Part model, mm, in its own coordinate system. A direction names the side the tool comes from. Coordinates: 2 decimals unless noted, no trailing zeros. Write each loop counter-clockwise with the first axis right and the second up, starting at its lowest first coordinate (ties: lowest second). Pieces come first, ordered by that corner, then holes. Notation, with made-up numbers: (63.25, 10.5) -> (112.25, 10.5) arc R22 ccw to (112.25, 32.5) -> close; hole circle Ø10 at (47.5, -6.5). An arc over 180 degrees is marked (long way). Write item = value, one per line.
from build123d import *

# Parameters (mm, degrees)
CROQUIS1_R              = 1
SALIENTE_EXTRUIR1_DEPTH = 3


with BuildPart() as part:
    # Croquis1 → Saliente-Extruir1 (new body)
    with BuildSketch(Plane(origin=(0, 0, 0), x_dir=(1, 0, 0), z_dir=(0, 1, 0))):
        with BuildLine():
            Line((-1.930199007, 22.227708448), (9.995007766, -0.44472952))
            Line((9.995007766, -0.44472952), (9.995007766, -23.778062853))
            Line((9.995007766, -23.778062853), (14.995007766, -30.44472952))
            Line((14.995007766, -30.44472952), (19.995007766, -30.44472952))
            Line((19.995007766, -30.44472952), (19.995007766, -20.44472952))
            Line((19.995007766, -20.44472952), (14.995007766, -13.778062853))
            Line((14.995007766, -13.778062853), (14.995007766, -3.222172626))
            Line((14.995007766, -3.222172626), (17.495007766, 1.777827374))
            Line((17.495007766, 1.777827374), (17.495007766, 6.777827374))
            Line((17.495007766, 6.777827374), (6.920214539, 26.882832512))
            ThreePointArc((6.920214539, 26.882832512), (0.167445734, 28.980477254), (-1.930199007, 22.227708448))
        make_face()
        with Locations((2.495007766, 24.55527048)):
            Circle(CROQUIS1_R, mode=Mode.SUBTRACT)
        with Locations((12.371532383, 5.777827374)):
            Circle(CROQUIS1_R, mode=Mode.SUBTRACT)
    extrude(amount=SALIENTE_EXTRUIR1_DEPTH)


solid = part.part
Q1. Saw through at D-D on x = 4.75. Give the cut face in (y, z), and give its area (3 significant figures).
Model answer:
outline = (0, -29.02) -> (3, -29.02) -> (3, -9.53) -> (0, -9.53) -> close
area = 58.5 mm²
Q2. Mould opens along Z. For faces 1 (the face through (12.28, 1.48, -16.69)), 2 (the face through (14.995, 1, 9)), 3 (the face through (11, 0, 0)) say: released by +Z, released by -Z, zero draft, split by the parting line, or undercut.
Model answer:
face_1 = released by -Z
face_2 = undercut
face_3 = zero draft
Q3. Saw through at C-C on z = 7. Give the cut face in (x, y) (3 decimals), and give its area (3 significant figures).
Model answer:
outline = (9.995, 0) -> (14.995, 0) -> (14.995, 3) -> (9.995, 3) -> close
area = 15.0 mm²
Q4. Which spindle directions (+Z, -Z, +X, -X, +Y, -Y) get a long thin tool onto all of the face, cutting with end or side? Do faces 4 (the face through (17.495, 1, -4)), 5 (the face through (16.228, 1.479, 0.757)), 6 (the face through (9.995, 1, 12)). Say none if no direction does.
Model answer:
face_4 = -Z, +X, +Y, -Y
face_5 = +X, +Y, -Y
face_6 = +Z, -X, +Y, -Y
Q5. Saw through at B-B on y = 2.1. Give the cut face in (x, z) (3 decimals), and give its area (3 significant figures).
Model answer:
outline = (-1.93, -22.228) arc R5 ccw to (6.92, -26.883) -> (17.495, -6.778) -> (17.495, -1.778) -> (14.995, 3.222) -> (14.995, 13.778) -> (19.995, 20.445) -> (19.995, 30.445) -> (14.995, 30.445) -> (9.995, 23.778) -> (9.995, 0.445) -> close; hole circle Ø2 at (2.495, -24.555); hole circle Ø2 at (12.372, -5.778)
area = 502 mm²
Q6. Saw through at A-A on x = 12.75. Give the cut face in (y, z), and give its area (3 significant figures).
Model answer:
outline = (0, -15.8) -> (3, -15.8) -> (3, -6.7) -> (0, -6.7) -> close; (0, -4.85) -> (3, -4.85) -> (3, 27.45) -> (0, 27.45) -> close
area = 124 mm²
Q7. Pin check, flat tips, straight feed: pin 1 (0.9 mm diameter, centred on y = 2, z = 7, fed in from -X) (3 decimals); pin 2 (1.5 mm diameter, centred on x = 1, y = 1.5, fed in from +Z); pin 3 (1.5 mm diameter, centred on y = 2, z = 8, fed in from +X) (3 decimals). Stop position of each tip, or through.
Model answer:
pin_1 = 9.995
pin_2 = -15.23
pin_3 = 14.995
Q8. Probe line 1 (X direction, y = 0.65, z = 6) (3 decimals); line 2 (Z direction, x = 3.25, y = 0.85); line 3 (X direction, y = 1.9, z = -5) (3 decimals). List the from-to ranges inside material, lowest first. Write a range as from..to.
Model answer:
line_1 = 9.995..14.995
line_2 = -29.5..-25.21, -23.9..-12.38
line_3 = 7.131..11.743, 13..17.495
